Here's how the part is built. I have some questions about the finished solid (model axes, mm). A direction names the side the tool comes from. Coordinates: 2 decimals unless noted, no trailing zeros. Write each loop counter-clockwise with the first axis right and the second up, starting at its lowest first coordinate (ties: lowest second). Pieces come first, ordered by that corner, then holes. Notation, with made-up numbers: (61, 74) -> (115, 74) arc R8 ccw to (115, 80) -> close; hole circle Ø5 at (9.25, 44). An arc over 180 degrees is marked (long way). Answer in a Markdown table with one row per item. Add a question column.
from build123d import *

# Parameters (mm, degrees)
BOSS_EXTRUDE1_DEPTH = 15
CUT_EXTRUDE1_REACH  = 7
SKETCH2_R           = 2.25
FILLET1_R           = 5


with BuildPart() as part:
    # Sketch1 → Boss-Extrude1 (new body)
    with BuildSketch(Plane.XY):
        with BuildLine():
            Line((0, 35), (0, 0))
            Line((0, 0), (20, 0))
            Line((20, 0), (20, 5))
            Line((20, 5), (10, 5))
            ThreePointArc((10, 5), (6.464466094, 6.464466094), (5, 10))
            Line((5, 10), (5, 33.75))
            ThreePointArc((5, 33.75), (4.633883476, 34.633883476), (3.75, 35))
            Line((3.75, 35), (0, 35))
        make_face()
    extrude(amount=BOSS_EXTRUDE1_DEPTH)

    # Sketch2 → Cut-Extrude1 (cut, up to next)
    with BuildSketch(Plane(origin=(0, 5, 0), x_dir=(1, 0, 0), z_dir=(0, 1, 0)), mode=Mode.PRIVATE) as cut_extrude1_sk1:
        with Locations((15, -7.5)):
            Circle(SKETCH2_R)
    cut_extrude1_tool1 = extrude(cut_extrude1_sk1.sketch, amount=-CUT_EXTRUDE1_REACH, mode=Mode.PRIVATE) & part.part
    add(cut_extrude1_tool1.solids().sort_by_distance((15, 5, 7.5))[0], mode=Mode.SUBTRACT)

    # Fillet1
    fillet1_edges = [part.edges().sort_by_distance(p)[0] for p in [
        (20, 2.5, 15),
        (20, 2.5, 0),
    ]]
    fillet(fillet1_edges, radius=FILLET1_R)


solid = part.part
Q1. For faces 5 (the flat face through (5, 22, 7)), 6 (the flat face through (4, 14, 15)), which set-ups out of +Z, -Z, +X, -X, +Y, -Y let a thin tool reach every point of the face, with its end or its side?
Q2. I need wall thicknesses on line 1 (X direction, y = 3, z = 7.5); line 2 (Z direction, x = 15, y = 3); line 3 (X direction, y = 26, z = 7). Which ranges of each line are inside material? Lowest first, please. Write a range as [from, to].
Q3. Imagine slicing it at A-A on x = 13.25. Please give me the cut outline in (y, z), plus the area to 3 significant figures.
Q4. If we mould it in two halves opening along Z, with no side actions, what happens to faces 1 (the cylindrical face through (7, 6, 7)), 2 (the cylindrical face through (18, 3, 1)), 3 (the cylindrical face through (18, 3, 14)), 4 (the cylindrical face through (16.21, 2.535, 5.603))? For each: pulls with the +Z half, pulls with the -Z half, needs draft (parallel to the pull), parting line crosses it, or undercut.
Q5. Imagine slicing it at B-B on z = 14. Please give me the cut outline in (x, y), plus the area to 3 significant figures.
Q6. Imagine slicing it at C-C on z = 8.75. Please give me the cut outline in (x, y), plus the area to 3 significant figures.
Q7. I'm going to push flat-ended pins straight in: P1, Ø3, axis at y = 10, z = 10.5, coming from the +X side; P2, Ø6, axis at x = 13.5, z = 13, coming from the +Y side; P3, Ø3, axis at x = 6, z = 12, coming from the +Y side; P4, Ø3.5, axis at x = 15, z = 7.5, coming from the +Y side. Where does each tip first touch, or does it pass through?
Q8. Imagine slicing it at D-D on y = 21. Please give me the cut outline in (x, z).
Result sheet:
| question | item | result |
|---|---|---|
| 1 | face 5 | +Z, -Z, +X, +Y |
| 1 | face 6 | +Z, +X, -X, +Y, -Y |
| 2 | line 1 | x = [0, 12.75], [17.25, 20] |
| 2 | line 2 | z = [0, 5.25], [9.75, 15] |
| 2 | line 3 | x = [0, 5] |
| 3 | outline | (0, 0) -> (5, 0) -> (5, 6.09) -> (0, 6.09) -> close; (0, 8.91) -> (5, 8.91) -> (5, 15) -> (0, 15) -> close |
| 3 | area | 60.9 mm^2 |
| 4 | face 1 | needs draft |
| 4 | face 2 | pulls with the -Z half |
| 4 | face 3 | pulls with the +Z half |
| 4 | face 4 | undercut |
| 5 | outline | (0, 0) -> (18, 0) -> (18, 5) -> (10, 5) arc R5 cw to (5, 10) -> (5, 33.75) arc R1.25 ccw to (3.75, 35) -> (0, 35) -> close |
| 5 | area | 245 mm^2 |
| 6 | outline | (0, 0) -> (13.13, 0) -> (13.13, 5) -> (10, 5) arc R5 cw to (5, 10) -> (5, 33.75) arc R1.25 ccw to (3.75, 35) -> (0, 35) -> close; (16.87, 0) -> (20, 0) -> (20, 5) -> (16.87, 5) -> close |
| 6 | area | 236 mm^2 |
| 7 | P1 | stops at x = 5.23 |
| 7 | P2 | stops at y = 5 |
| 7 | P3 | stops at y = 34.75 |
| 7 | P4 | passes through |
| 8 | outline | (0, 0) -> (5, 0) -> (5, 15) -> (0, 15) -> close |
